The model under review builds one solid part; all positions refer to its coordinate system, in mm. Face numbers are marked on the shaded views. A direction names the side the tool comes from. Coordinates: 2 decimals unless noted, no trailing zeros. Write each loop counter-clockwise with the first axis right and the second up, starting at its lowest first coordinate (ties: lowest second). Pieces come first, ordered by that corner, then holes.
1) Add section B-B, the plane x = 50. State the section outline as (y, z) points.
2) Add section A-A, the plane z = -94. State the section outline as (x, y) points.
3) Add section D-D, the plane x = 295. State the section outline as (y, z) points, then the cut area to 3 significant figures.
4) For line 1 (X direction, y = 10.25, z = -35); line 2 (X direction, y = 62, z = -145.5); line 3 (Y direction, x = 389.5, z = -94), list the stretches that pass through material, from the lowest coordinate up.
5) Machinability: for the marked faces 1, 2 and 3, which of the approach directions +Z, -Z, +X, -X, +Y, -Y give a long, thin tool a straight path to every point of the face, cutting with its end or side? Answer none if there is none.
6) For P1, Ø2, axis at x = 63, z = -46.5, coming from the +Y side; P2, Ø4, axis at x = 168, y = 30.5, coming from the -Z side; P3, Ø3, axis at x = 149.5, z = -75.5, coming from the +Y side, all flat-tipped, find the tip position at first contact; note any pin that passes through.
7) Mouldability with a two-part tool opening along X and no side actions: class the marked faces 4, 5, 6 and 7 as released by +X, released by -X, zero draft, split by the parting line, or undercut.
8) Add section C-C, the plane y = 195. State the section outline as (x, z) points, then the cut area to 3 significant figures.
from build123d import *

# Parameters (mm, degrees)
SKETCH_1_W      = 400
SKETCH_1_H      = 165
SKETCH_1_R      = 13
EXTRUDE_1_DEPTH = 16
SKETCH_2_W      = 368
SKETCH_2_H      = 10
EXTRUDE_2_DEPTH = 125
SKETCH_3_R      = 20.5
EXTRUDE_3_DEPTH = 16


with BuildPart() as part:
    # 草图1 → 凸台-拉伸1 (new body)
    with BuildSketch(Plane(origin=(0, 0, 0), x_dir=(1, 0, 0), z_dir=(0, 1, 0))):
        with Locations((200, 82.5)):
            Rectangle(SKETCH_1_W, SKETCH_1_H)
        with Locations(Location((350, 115, 0), (0, 0, 270))):
            Circle(SKETCH_1_R, mode=Mode.SUBTRACT)
        with Locations(Location((50, 115, 0), (0, 0, 270))):
            Circle(SKETCH_1_R, mode=Mode.SUBTRACT)
        with Locations(Location((50, 35, 0), (0, 0, 270))):
            Circle(SKETCH_1_R, mode=Mode.SUBTRACT)
        with Locations(Location((350, 35, 0), (0, 0, 270))):
            Circle(SKETCH_1_R, mode=Mode.SUBTRACT)
    extrude(amount=EXTRUDE_1_DEPTH)

    # 草图2 → 凸台-拉伸2 (add)
    with BuildSketch(Plane(origin=(0, 16, 0), x_dir=(1, 0, 0), z_dir=(0, 1, 0))):
        with Locations((200, 75)):
            Rectangle(SKETCH_2_W, SKETCH_2_H)
    extrude(amount=EXTRUDE_2_DEPTH)

    # 草图3 → 凸台-拉伸3 (add)
    with BuildSketch(Plane(origin=(384, 0, 0), x_dir=(0, 0, -1), z_dir=(1, 0, 0))):
        with BuildLine():
            Line((165, 16), (165, 26))
            Line((165, 26), (148.762358111, 200.107262875))
            ThreePointArc((148.762358111, 200.107262875), (97.468660954, 249.890512761), (40.316177192, 206.960232804))
            Line((40.316177192, 206.960232804), (0, 26))
            Line((0, 26), (0, 16))
            Line((0, 16), (165, 16))
        make_face()
        with Locations((94, 195)):
            Circle(SKETCH_3_R, mode=Mode.SUBTRACT)
    extrude_3 = extrude(amount=EXTRUDE_3_DEPTH)

    # 镜向1: 凸台-拉伸3 across plane
    add(extrude_3.mirror(Plane(origin=(200, 0, 0), x_dir=(0, 0, 1), z_dir=(1, 0, 0))))


solid = part.part
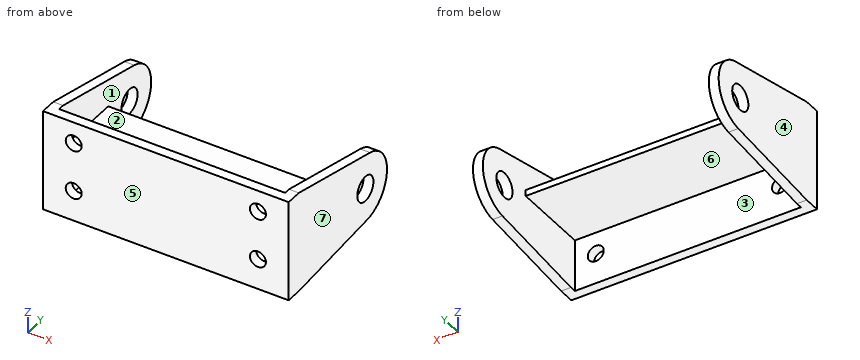
Geometry results:
1. outline: (0, -165) - (16, -165) - (16, -128) - (0, -128) - close; (0, -102) - (16, -102) - (16, -80) - (141, -80) - (141, -70) - (16, -70) - (16, -48) - (0, -48) - close; (0, -22) - (16, -22) - (16, 0) - (0, 0) - close
2. outline: (0, 0) - (400, 0) - (400, 174.5) - (384, 174.5) - (384, 16) - (16, 16) - (16, 174.5) - (0, 174.5) - close; (0, 215.5) - (16, 215.5) - (16, 250) - (0, 250) - close; (384, 215.5) - (400, 215.5) - (400, 250) - (384, 250) - close
3. outline: (0, -165) - (16, -165) - (16, -80) - (141, -80) - (141, -70) - (16, -70) - (16, 0) - (0, 0) - close
3. area: 3,890 mm2
4. line 1: x = 0 to 37, 63 to 337, 363 to 400
4. line 2: x = 0 to 16, 384 to 400
4. line 3: y = 0 to 174.5, 215.5 to 250
5. face 1: +Y
5. face 2: +Z, +Y
5. face 3: -Z, +Y
6. P1: stops at y = 16
6. P2: stops at z = -80
6. P3: stops at y = 141
7. face 4: released by -X
7. face 5: zero draft
7. face 6: undercut
7. face 7: released by +X
8. outline: (0, -149.24) - (16, -149.24) - (16, -114.5) - (0, -114.5) - close; (0, -73.5) - (16, -73.5) - (16, -37.65) - (0, -37.65) - close; (384, -149.24) - (400, -149.24) - (400, -114.5) - (384, -114.5) - close; (384, -73.5) - (400, -73.5) - (400, -37.65) - (384, -37.65) - close
8. area: 2,260 mm2
